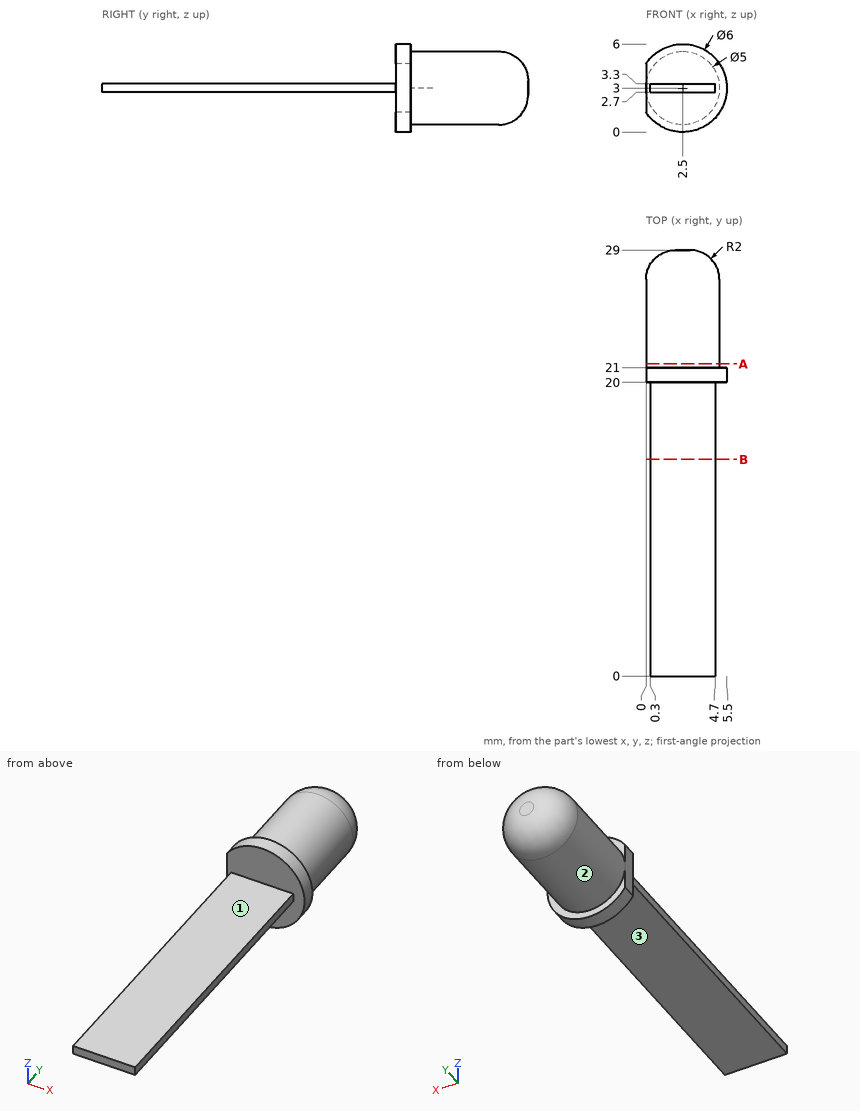
Here's the drawing with two shaded views (mm, measured from the low corner). I have some questions. A direction names the side the tool comes from. Coordinates: 2 decimals unless noted, no trailing zeros. Order: outer loops, then holes, each group sorted by start corner. A loop starts at its lowest first (then second) coordinate and runs counter-clockwise, first axis right, second up. Notation, with made-up numbers: M 15.25,61.25 L 20.25,61.25 A22 cw 20.25,99.25 Z; hole C 24,28 d10. An arc over 180 degrees is marked long. Answer as CSV lines item,"result".
Item 1: Imagine slicing it at B-B on y = 14.75. Write out the boundary of the cut face in (x, z).
Results found:
outline,"M 0.3,2.7 L 4.7,2.7 L 4.7,3.3 L 0.3,3.3 Z"
Item 2: For pin 1 (1.5 mm diameter, centred on y = 23.5, z = 1, fed in from -X); pin 2 (1 mm diameter, centred on x = 4.5, y = 23.5, fed in from -Z); pin 3 (1.5 mm diameter, centred on x = 4.5, y = 4, fed in from +Z), each with a flat end and sliding along its axis, tell me the tip position at first contact or that it passes through.
Results found:
pin 1,"x = 0.33"
pin 2,"z = 1"
pin 3,"z = 3.3"
Item 3: Imagine slicing it at A-A on y = 21.25. Write out the boundary of the cut face in (x, z).
Results found:
outline,"C 2.5,3 d5"
Item 4: If I drill on line 1 (Z direction, x = 2.8, y = 18); line 2 (Y direction, x = 1.4, z = 5.75); line 3 (Z direction, x = 2.6, y = 20.5), over which ranges is the centre line in solid material (lowest first)?
Results found:
line 1,"2.7 to 3.3"
line 2,"20 to 21"
line 3,"0 to 6"
Item 5: On a 3-axis mill with a long thin cutter (end or side, diameter ignored), from which of +Z, -Z, +X, -X, +Y, -Y can I reach the whole of each face in a straight line? I mean the marked faces 1, 2 and 3. Say none if no direction works.
Results found:
face 1,"+Z, +X, -X, -Y"
face 2,"+Y"
face 3,"-Z, +X, -X, -Y"
